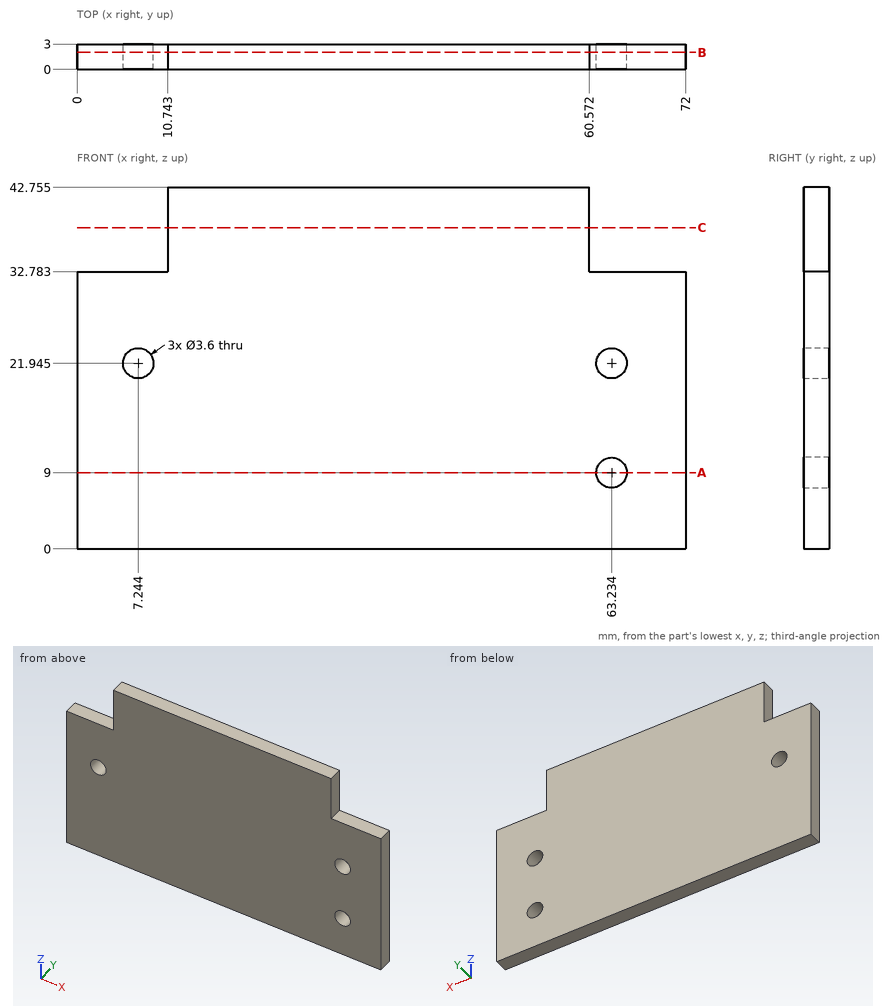
Can you work these out from the drawing? Everything is in mm from the part's minimum corner. Round coordinates to 2 decimals unless told otherwise and drop trailing zeros. Write each loop counter-clockwise with the first axis right and the second up, starting at its lowest first coordinate (ties: lowest second). Pieces come first, ordered by that corner, then holes. Notation, with made-up numbers: (25, 39.25) - (75, 39.25) arc R17 cw to (75, 55.25) - close; hole circle Ø10 at (57, 62.25). An arc over 180 degrees is marked (long way). Put each result on its own line as item: value. Start each with the question number.
(1) I want a section at C-C, the plane z = 38. Please give me the cut outline in (x, y).
(2) I want a section at B-B, the plane y = 2. Please give me the cut outline in (x, z) (1 decimal).
(3) Will this pin go through, and if not, where does the flat tip stop? pin 1 (0.9 mm diameter, centred on y = 1.5, z = 36.5, fed in from -X).
(4) I want a section at A-A, the plane z = 9. Please give me the cut outline in (x, y) (1 decimal).
(5) I need wall thicknesses on probe 1 along Z at (x, y) = (63, 0.95) (1 decimal); probe 2 along X at (y, z) = (1, 21) (1 decimal); probe 3 along X at (y, z) = (0.1, 9) (1 decimal). Which ranges of each line are inside material? Lowest first, please.
Here are the results:
1. outline: (10.74, 0) - (60.57, 0) - (60.57, 3) - (10.74, 3) - close
2. outline: (0, 0) - (72, 0) - (72, 32.8) - (60.6, 32.8) - (60.6, 42.8) - (10.7, 42.8) - (10.7, 32.8) - (0, 32.8) - close; hole circle Ø3.6 at (7.2, 21.9); hole circle Ø3.6 at (63.2, 9); hole circle Ø3.6 at (63.2, 21.9)
3. pin 1: stops at x = 10.74
4. outline: (0, 0) - (61.4, 0) - (61.4, 3) - (0, 3) - close; (65, 0) - (72, 0) - (72, 3) - (65, 3) - close
5. probe 1: z = 0 to 7.2, 10.8 to 20.2, 23.7 to 32.8
5. probe 2: x = 0 to 5.7, 8.8 to 61.7, 64.8 to 72
5. probe 3: x = 0 to 61.4, 65 to 72
